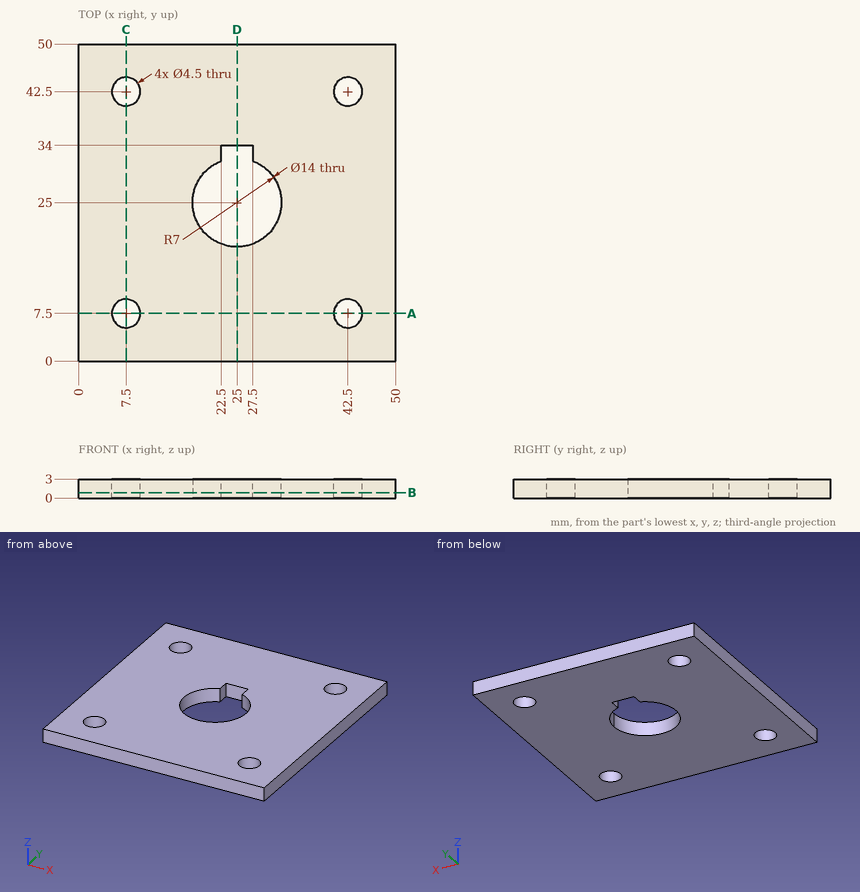
Check sheet for the drawn part. Datum: minimum x, y, z corner. Units: mm. Give positions to 0.01 mm unless a question says otherwise; leave off trailing zeros. Loops run counter-clockwise (first coordinate to the right, second up) from the corner with the lowest first, then second, coordinate; pieces in that order, holes last. Notation, with made-up numbers: M 84,29.5 L 143,29.5 A10 ccw 143,46.5 Z; hole C 63,77 d6. An arc over 180 degrees is marked long. Return JSON: item names as keys, results as strings.
1) Section check A-A, the plane y = 7.5. Enter the section's corners in (x, z), and give its area (3 significant figures).
Findings:
{"outline": "M 0,0 L 5.25,0 L 5.25,3 L 0,3 Z; M 9.75,0 L 40.25,0 L 40.25,3 L 9.75,3 Z; M 44.75,0 L 50,0 L 50,3 L 44.75,3 Z", "area": "123 mm2"}
2) Section check B-B, the plane z = 0.85. Enter the section's corners in (x, y), and give its area (3 significant figures).
Findings:
{"outline": "M 0,0 L 50,0 L 50,50 L 0,50 Z; hole C 7.5,7.5 d4.5; hole C 7.5,42.5 d4.5; hole M 22.5,31.54 A7 ccw long 27.5,31.54 L 27.5,34 L 22.5,34 Z; hole C 42.5,7.5 d4.5; hole C 42.5,42.5 d4.5", "area": "2,270 mm2"}
3) Section check D-D, the plane x = 25. Enter the section's corners in (y, z).
Findings:
{"outline": "M 0,0 L 18,0 L 18,3 L 0,3 Z; M 34,0 L 50,0 L 50,3 L 34,3 Z"}
4) Gauge pin test, flat end, axial feed: P1, Ø4, axis at x = 42.5, y = 7.5, coming from the -Z side. Record the tip position at first contact, or that the pin passes through.
Findings:
{"P1": "passes through"}
5) Material ranges on L1, parallel to Y at x = 7.5, z = 1.2; L2, parallel to X at y = 44, z = 2.7, recorded low to high. Write a range as [from, to].
Findings:
{"L1": "y = [0, 5.25], [9.75, 40.25], [44.75, 50]", "L2": "x = [0, 5.82], [9.18, 40.82], [44.18, 50]"}
